Work out the finished part from the listing and answer in its coordinate system (mm). Face numbers are marked on the shaded views. Round coordinates to 2 decimals unless told otherwise and drop trailing zeros. Loops run counter-clockwise (first coordinate to the right, second up) from the corner with the lowest first, then second, coordinate; pieces in that order, holes last. Notation, with made-up numbers: M 89,53.25 L 97,53.25 A18 cw 97,66.25 Z; hole C 0.5,53.25 d3. An arc over 180 degrees is marked long. One line per item, written item: value.
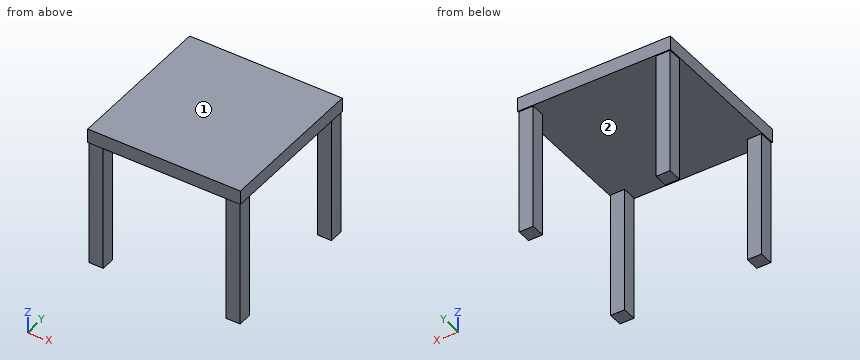
```python
from build123d import *

# Parameters (mm, degrees)
F1_W     = 50.8
F1_H     = 50.8
F2_DEPTH = 508
F5_W     = 50.8
F5_H     = 50.8
F6_DEPTH = 50.8
F8_W     = 552.45
F8_H     = 552.45
F8_W_2   = 546.1
F8_H_2   = 546.1
F9_DEPTH = 50.8


with BuildPart() as f2:
    # F1 (on Top) → F2 (new body)
    with BuildSketch(Plane.XY):
        with Locations((-247.65, 247.65)):
            Rectangle(F1_W, F1_H)
    extrude(amount=F2_DEPTH)


with BuildPart() as f3_1:
    # F3: instance of F2
    add(f2.part.mirror(Plane.YZ))


with BuildPart() as f4_1:
    # F4: instance of F2
    add(f2.part.mirror(Plane.XZ))


with BuildPart() as f4_2:
    # F4: instance of F3_1
    add(f3_1.part.mirror(Plane.XZ))


with BuildPart() as f6:
    # F5 (on face) → F6 (new body)
    with BuildSketch(Plane.XY.offset(508)):
        Polygon((-273.05, 222.25), (-273.05, -273.05), (273.05, -273.05), (273.05, 273.05), (-222.25, 273.05), (-222.25, 222.25), align=None)
        with Locations((-247.65, 247.65)):
            Rectangle(F5_W, F5_H)
    extrude(amount=-F6_DEPTH)


with BuildPart() as f2_1:
    add(f2.part)

    # F7: union F6, F3_1, F4_1, F4_2
    add(f6.part)
    add(f3_1.part)
    add(f4_1.part)
    add(f4_2.part)

    # F8 (on face) → F9 (join, through all)
    with BuildSketch(Plane.XY.offset(508)):
        Rectangle(F8_W, F8_H)
        Rectangle(F8_W_2, F8_H_2, mode=Mode.SUBTRACT)
    extrude(amount=-F9_DEPTH)


solid = f2_1.part
```
1) Find section D-D (x = -174). Give the vertices of the cut face in (y, z) (3 decimals), then the cut area to 3 significant figures.
Check values:
outline: M -276.225,457.2 L 276.225,457.2 L 276.225,508 L -276.225,508 Z
area: 28,100 mm2
2) Find the intervals of material crossed by probe 1 along X at (y, z) = (251, 244.5); probe 2 along Z at (x, y) = (-7.5, 129.5), in increasing order. Write a range as from..to.
Check values:
probe 1: -273.05..-222.25, 222.25..273.05
probe 2: 457.2..508
3) Find section A-A (z = 135). Give the vertices of the cut face in (x, y).
Check values:
outline: M -273.05,-273.05 L -222.25,-273.05 L -222.25,-222.25 L -273.05,-222.25 Z; M -273.05,222.25 L -222.25,222.25 L -222.25,273.05 L -273.05,273.05 Z; M 222.25,-273.05 L 273.05,-273.05 L 273.05,-222.25 L 222.25,-222.25 Z; M 222.25,222.25 L 273.05,222.25 L 273.05,273.05 L 222.25,273.05 Z
4) This flat-tipped pin is pushed along its axis until it touches: pin 1 (12 mm diameter, centred on x = 122.5, y = -105.5, fed in from -Z). Where does it stop, or does it pass through?
Check values:
pin 1: z = 457.2
5) Find section B-B (y = 236). Give the vertices of the cut face in (x, z) (3 decimals), then the cut area to 3 significant figures.
Check values:
outline: M -276.225,457.2 L -273.05,457.2 L -273.05,0 L -222.25,0 L -222.25,457.2 L 222.25,457.2 L 222.25,0 L 273.05,0 L 273.05,457.2 L 276.225,457.2 L 276.225,508 L -276.225,508 Z
area: 74,500 mm2
6) The mould has two halves that part along X. Classify the marked faces 1 and 2: +X half, -X half, draft (parallel to the pull), parting line (faces both ways), or undercut.
Check values:
face 1: draft
face 2: undercut
